from build123d import *

# Parameters (mm, degrees)
SKETCH1_R           = 5
BOSS_EXTRUDE1_DEPTH = 11.5
FILLET1_R           = 5
SKETCH4_W           = 4.6
SKETCH4_H           = 15
CUT_EXTRUDE1_DEPTH  = 2
CHAMFER1_SIZE       = 0.2


with BuildPart() as part:
    # Sketch1 → Boss-Extrude1 (new body)
    with BuildSketch(Plane.XY):
        Circle(SKETCH1_R)
    extrude(amount=BOSS_EXTRUDE1_DEPTH)

    # Fillet1
    fillet1_edges = [part.edges().sort_by_distance(p)[0] for p in [
        (-5, 0, 11.5),
    ]]
    fillet(fillet1_edges, radius=FILLET1_R)

    # Sketch4 → Cut-Extrude1 (cut)
    with BuildSketch(Plane(origin=(0, 0, 0), x_dir=(-1, 0, 0), z_dir=(0, 0, -1))):
        Rectangle(SKETCH4_W, SKETCH4_H)
    extrude(amount=-CUT_EXTRUDE1_DEPTH, mode=Mode.SUBTRACT)

    # Chamfer1
    chamfer1_edges = [part.edges().sort_by_distance(p)[0] for p in [
        (-5, 0, 0),
        (4.272001873, 2.598076211, 0),
        (-2.3, 0, 0),
        (2.3, 0, 0),
    ]]
    chamfer(chamfer1_edges, length=CHAMFER1_SIZE)


solid = part.part
Could you check a few things on this model? Use its own coordinates, in mm. A direction names the side the tool comes from. Give positions to 0.01 mm unless a question says otherwise; leave off trailing zeros. Write each loop counter-clockwise with the first axis right and the second up, starting at its lowest first coordinate (ties: lowest second). Pieces come first, ordered by that corner, then holes. Notation, with made-up numbers: (-3.75, 51.5) - (50.25, 51.5) arc R19 cw to (50.25, 65.5) - close; hole circle Ø3 at (1.5, 17). An arc over 180 degrees is marked (long way). Use CSV: the item, a comma, the result in double quotes. Start each with the question number.
Item 1: I want a section at B-B, the plane x = 0. Please give me the cut outline in (y, z), then the cut area to 3 significant figures.
Item 2: I want a section at A-A, the plane y = 0. Please give me the cut outline in (x, z), then the cut area to 3 significant figures.
Item 3: I want a section at C-C, the plane z = 5.75. Please give me the cut outline in (x, y).
Item 4: If I drill on line 1 along X through (y, z) = (2.75, 1.25); line 2 along Z through (x, y) = (-3.25, 0.25); line 3 along Y through (x, z) = (0.5, 5.75), over which ranges is the centre line in solid material (lowest first)?
Item 5: I want a section at D-D, the plane z = 7.75. Please give me the cut outline in (x, y), then the cut area to 3 significant figures.
Item 6: For faces 1 (the face through (2.3, 0, 1)), 2 (the face through (-3, 0, 0)), which set-ups out of +Z, -Z, +X, -X, +Y, -Y let a thin tool reach every point of the face, with its end or its side?
Item 7: I'm going to push flat-ended pins straight in: pin 1 (4 mm diameter, centred on x = -2.5, z = 5, fed in from +Y); pin 2 (0.9 mm diameter, centred on y = -2, z = 1, fed in from +X); pin 3 (1 mm diameter, centred on x = -2, y = -3, fed in from +Z). Where does each tip first touch, or does it pass through?
Item 8: If we mould it in two halves opening along X, with no side actions, what happens to faces 3 (the face through (0, 0, 2)), 4 (the face through (3, 0, 0)), 5 (the face through (4.619, -1.915, 3.306))? For each: pulls with the +X half, pulls with the -X half, needs draft (parallel to the pull), parting line crosses it, or undercut.
Findings:
1,outline,"(-5, 2) - (5, 2) - (5, 6.5) arc R5 ccw to (-5, 6.5) - close"
1,area,"84.3 mm2"
2,outline,"(-5, 0.2) - (-4.8, 0) - (-2.5, 0) - (-2.3, 0.2) - (-2.3, 2) - (2.3, 2) - (2.3, 0.2) - (2.5, 0) - (4.8, 0) - (5, 0.2) - (5, 6.5) arc R5 ccw to (-5, 6.5) - close"
2,area,"95.0 mm2"
3,outline,"circle Ø10 at (0, 0)"
4,line 1,"x = -4.18 to -2.3, 2.3 to 4.18"
4,line 2,"z = 0 to 10.29"
4,line 3,"y = -4.97 to 4.97"
5,outline,"circle Ø9.68 at (0, 0)"
5,area,"73.6 mm2"
6,face 1,"-Z, +Y, -Y"
6,face 2,"-Z, +X, -X, +Y, -Y"
7,pin 1,"stops at y = 4.97"
7,pin 2,"stops at x = 4.75"
7,pin 3,"stops at z = 10.42"
8,face 3,"undercut"
8,face 4,"needs draft"
8,face 5,"parting line crosses it"
